Check sheet for the modelled part. Datum: model origin and axes. Units: mm. Face numbers are marked on the shaded views. A direction names the side the tool comes from. Round coordinates to 2 decimals unless told otherwise and drop trailing zeros. Write each loop counter-clockwise with the first axis right and the second up, starting at its lowest first coordinate (ties: lowest second). Pieces come first, ordered by that corner, then holes. Notation, with made-up numbers: (64, 42) -> (71, 42) arc R25 ccw to (71, 76) -> close; hole circle Ø2 at (-6.75, 49). An arc over 180 degrees is marked (long way). Answer as a JSON object with one key per item and string values. Group by question number.
```python
from build123d import *

# Parameters (mm, degrees)
SKETCH1_W           = 50
SKETCH1_H           = 30
SKETCH1_R           = 2.6
BOSS_EXTRUDE1_DEPTH = 7
FILLET1_R           = 10
SKETCH2_R           = 4.3
CUT_EXTRUDE1_DEPTH  = 4


with BuildPart() as part:
    # Sketch1 → Boss-Extrude1 (new body)
    with BuildSketch(Plane(origin=(0, 0, 0), x_dir=(1, 0, 0), z_dir=(0, 1, 0))):
        with Locations((25, 15)):
            Rectangle(SKETCH1_W, SKETCH1_H)
        with Locations(Location((25, 25, 0), (0, 0, 270))):
            Circle(SKETCH1_R, mode=Mode.SUBTRACT)
        with Locations(Location((25, 5, 0), (0, 0, 270))):
            Circle(SKETCH1_R, mode=Mode.SUBTRACT)
    extrude(amount=BOSS_EXTRUDE1_DEPTH)

    # Fillet1
    fillet1_edges = [part.edges().sort_by_distance(p)[0] for p in [
        (0, 3.5, -30),
        (50, 3.5, -30),
        (50, 3.5, 0),
        (0, 3.5, 0),
    ]]
    fillet(fillet1_edges, radius=FILLET1_R)

    # Sketch2 → Cut-Extrude1 (cut)
    with BuildSketch(Plane(origin=(0, 7, 0), x_dir=(1, 0, 0), z_dir=(0, 1, 0))):
        with Locations(Location((25, 25, 0), (0, 0, 270))):
            Circle(SKETCH2_R)
        with Locations(Location((25, 5, 0), (0, 0, 270))):
            Circle(SKETCH2_R)
    extrude(amount=-CUT_EXTRUDE1_DEPTH, mode=Mode.SUBTRACT)


solid = part.part
```
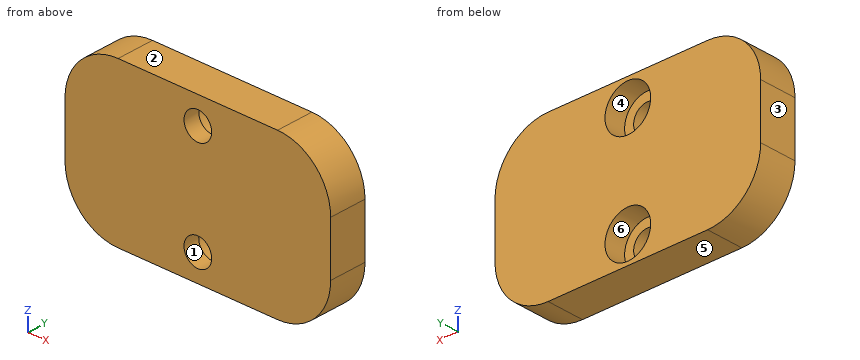
(1) Release check for a two-part mould opening along X. For the marked faces 1, 2, 3 and 4 record: pulls with the +X half, pulls with the -X half, needs draft (parallel to the pull), parting line crosses it, or undercut.
(2) Access from +Z, -Z, +X, -X, +Y, -Y to the whole of each face (thin tool, end or side, straight path). Record for the marked faces 5 and 6.
(3) Scan lines: line 1 along Z through (x, y) = (25, 0.8); line 2 along Y through (x, z) = (29, -4.5); line 3 along X through (y, z) = (5.8, -5). Record each from-to range of solid material in increasing order.
(4) Section check C-C on z = -25. Record the cut outline in (x, y), then the cut area to 3 significant figures.
(5) Section check B-B on y = 4.75. Record the cut outline in (x, z), then the cut area to 3 significant figures.
(6) Section check D-D on y = 0.5. Record the cut outline in (x, z).
(7) Go/stop test with flat-tipped pins: pin 1 Ø9.5 at (x, z) = (24.5, -23) entering from +Y; pin 2 Ø7 at (x, z) = (25, -5) entering from +Y. Record where each tip stops, or that it passes through.
(8) Section check A-A on x = 25. Record the cut outline in (y, z), then the cut area to 3 significant figures.
Data:
{
 "1": {"face 1": "undercut", "face 2": "needs draft", "face 3": "pulls with the -X half", "face 4": "undercut"},
 "2": {"face 5": "-Z, +X, -X, +Y, -Y", "face 6": "+Y"},
 "3": {"line 1": "z = -30 to -27.6, -22.4 to -7.6, -2.4 to 0", "line 2": "y = 0 to 3", "line 3": "x = 1.34 to 20.7, 29.3 to 48.66"},
 "4": {"outline": "(1.34, 0) -> (22.4, 0) -> (22.4, 3) -> (20.7, 3) -> (20.7, 7) -> (1.34, 7) -> close; (27.6, 0) -> (48.66, 0) -> (48.66, 7) -> (29.3, 7) -> (29.3, 3) -> (27.6, 3) -> close", "area": "281 mm²"},
 "5": {"outline": "(0, -20) arc R10 ccw to (10, -30) -> (40, -30) arc R10 ccw to (50, -20) -> (50, -10) arc R10 ccw to (40, 0) -> (10, 0) arc R10 ccw to (0, -10) -> close; hole circle Ø8.6 at (25, -25); hole circle Ø8.6 at (25, -5)", "area": "1,300 mm²"},
 "6": {"outline": "(0, -20) arc R10 ccw to (10, -30) -> (40, -30) arc R10 ccw to (50, -20) -> (50, -10) arc R10 ccw to (40, 0) -> (10, 0) arc R10 ccw to (0, -10) -> close; hole circle Ø5.2 at (25, -25); hole circle Ø5.2 at (25, -5)"},
 "7": {"pin 1": "stops at y = 7", "pin 2": "stops at y = 3"},
 "8": {"outline": "(0, -30) -> (7, -30) -> (7, -29.3) -> (3, -29.3) -> (3, -27.6) -> (0, -27.6) -> close; (0, -22.4) -> (3, -22.4) -> (3, -20.7) -> (7, -20.7) -> (7, -9.3) -> (3, -9.3) -> (3, -7.6) -> (0, -7.6) -> close; (0, -2.4) -> (3, -2.4) -> (3, -0.7) -> (7, -0.7) -> (7, 0) -> (0, 0) -> close", "area": "110 mm²"}
}
